from build123d import *

# Parameters (mm, degrees)
SKETCH_1_W          = 20
SKETCH_1_H          = 15
EXTRUDE_1_DEPTH     = 70
SKETCH_2_R          = 4.25
CUT_EXTRUDE_1_DEPTH = 75.330343737
SKETCH_3_R          = 1.575
CUT_EXTRUDE_2_DEPTH = 75.330343737


with BuildPart() as part:
    # 草图1 → 凸台-拉伸1 (new body)
    with BuildSketch(Plane.XY):
        with Locations((10, -7.5)):
            Rectangle(SKETCH_1_W, SKETCH_1_H)
    extrude(amount=EXTRUDE_1_DEPTH)

    # 草图2 → 切除-拉伸1 (cut, through all)
    with BuildSketch(Plane(origin=(0, 0, 0), x_dir=(-1, 0, 0), z_dir=(0, 0, -1))):
        with Locations((-10, -7.5)):
            Circle(SKETCH_2_R)
    extrude(amount=-CUT_EXTRUDE_1_DEPTH, mode=Mode.SUBTRACT)

    # 草图3 → 切除-拉伸2 (cut, through all)
    with BuildSketch(Plane(origin=(20, 0, 0), x_dir=(0, 0, -1), z_dir=(1, 0, 0))):
        with Locations(Location((-60, -7.5, 0), (0, 0, 90))):
            Circle(SKETCH_3_R)
        with Locations(Location((-35, -7.5, 0), (0, 0, 90))):
            Circle(SKETCH_3_R)
        with Locations(Location((-10, -7.5, 0), (0, 0, 90))):
            Circle(SKETCH_3_R)
    extrude(amount=-CUT_EXTRUDE_2_DEPTH, mode=Mode.SUBTRACT)


solid = part.part
Here's how the part is built. I have some questions about the finished solid (model axes, mm). Coordinates: 2 decimals unless noted, no trailing zeros. Loops run counter-clockwise (first coordinate to the right, second up) from the corner with the lowest first, then second, coordinate; pieces in that order, holes last.
1. I need wall thicknesses on L1, parallel to Z at x = 16.75, y = -7.5 (3 decimals); L2, parallel to Y at x = 17.75, z = 35 (3 decimals); L3, parallel to X at y = -11, z = 35. Which ranges of each line are inside material? Lowest first, please.
2. Imagine slicing it at D-D, the plane x = 10. Please give me the cut outline in (y, z), and give its area (3 significant figures).
3. Imagine slicing it at A-A, the plane y = -7.5. Count the separate pieces of the cut face and the enclosed holes in it, and give its area (3 significant figures).
4. For P1, Ø3, axis at x = 4, y = -4.5, coming from the -Z side; P2, Ø5, axis at x = 9, y = -6.5, coming from the +Z side, each with a flat end and sliding along its axis, tell me the tip position at first contact or that it passes through.
5. Imagine slicing it at B-B, the plane x = 17.75. Please give me the cut outline in (y, z) (3 decimals).
6. If we mould it in two halves opening along Y, with no side actions, what happens to faces 1 (the flat face through (5, -7, 0)), 2 (the cylindrical face through (3.069, -7.841, 8.462)), 3 (the flat face through (10, 0, 35))? For each: pulls with the +Y half, pulls with the -Y half, needs draft (parallel to the pull), parting line crosses it, or undercut.
7. Imagine slicing it at C-C, the plane z = 10. Please give me the cut outline in (x, y) (3 decimals), and give its area (3 significant figures).
Taken from the geometry:
1. L1: z = 0 to 8.425, 11.575 to 33.425, 36.575 to 58.425, 61.575 to 70
1. L2: y = -15 to -9.075, -5.925 to 0
1. L3: x = 0 to 7.59, 12.41 to 20
2. outline: (-15, 0) - (-11.75, 0) - (-11.75, 70) - (-15, 70) - close; (-3.25, 0) - (0, 0) - (0, 70) - (-3.25, 70) - close
2. area: 455 mm2
3. separate pieces: 8
3. enclosed holes: 0
3. area: 696 mm2
4. P1: stops at z = 0
4. P2: passes through
5. outline: (-15, 0) - (0, 0) - (0, 70) - (-15, 70) - close; hole circle Ø3.15 at (-7.5, 10); hole circle Ø3.15 at (-7.5, 35); hole circle Ø3.15 at (-7.5, 60)
6. face 1: needs draft
6. face 2: undercut
6. face 3: pulls with the +Y half
7. outline: (0, -15) - (20, -15) - (20, -9.075) - (13.947, -9.075) arc R4.25 cw to (6.053, -9.075) - (0, -9.075) - close; (0, -5.925) - (6.053, -5.925) arc R4.25 cw to (13.947, -5.925) - (20, -5.925) - (20, 0) - (0, 0) - close
7. area: 206 mm2
